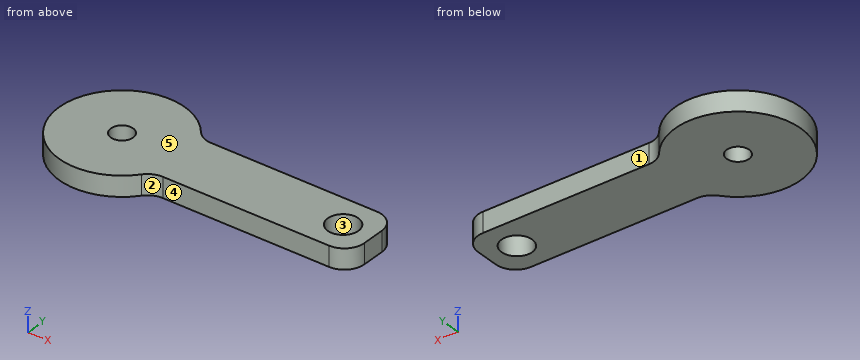
from build123d import *

# Parameters (mm, degrees)
BOSS_EXTRUDE1_DEPTH   = 1.6002
F_0_CLEARANCE_HOLE1_D = 1.778
F_2_CLEARANCE_HOLE1_D = 2.4384


with BuildPart() as part:
    # Sketch1 → Boss-Extrude1 (new body)
    with BuildSketch(Plane.XY):
        with BuildLine():
            Line((5.16599458, -2.5), (18.4125, -2.5))
            ThreePointArc((18.4125, -2.5), (19.535032015, -2.035032015), (20, -0.9125))
            Line((20, -0.9125), (20, 0.9125))
            ThreePointArc((20, 0.9125), (19.535032015, 2.035032015), (18.4125, 2.5))
            Line((18.4125, 2.5), (5.16599458, 2.5))
            ThreePointArc((5.16599458, 2.5), (4.474468718, 2.658532459), (3.921058505, 3.102466793))
            ThreePointArc((3.921058505, 3.102466793), (-5, 0), (3.921058505, -3.102466793))
            ThreePointArc((3.921058505, -3.102466793), (4.474468718, -2.658532459), (5.16599458, -2.5))
        make_face()
    extrude(amount=BOSS_EXTRUDE1_DEPTH)

    # #0 Clearance Hole1 (through all)
    with Locations(Plane.XY.offset(1.6002)):
        with Locations((0, 0)):
            Hole(F_0_CLEARANCE_HOLE1_D / 2)

    # #2 Clearance Hole1 (through all)
    with Locations(Plane.XY.offset(1.6002)):
        with Locations((17.615594793, 0)):
            Hole(F_2_CLEARANCE_HOLE1_D / 2)


solid = part.part
Could you check a few things on this model? Use its own coordinates, in mm. Face numbers are marked on the shaded views. A direction names the side the tool comes from. Give positions to 0.01 mm unless a question says otherwise; leave off trailing zeros. Write each loop counter-clockwise with the first axis right and the second up, starting at its lowest first coordinate (ties: lowest second). Pieces come first, ordered by that corner, then holes. Notation, with made-up numbers: (40, 82.25) - (67, 82.25) arc R15 ccw to (67, 93.25) - close; hole circle Ø10 at (9, 45). An arc over 180 degrees is marked (long way). Use CSV: the item, a comma, the result in double quotes. Start each with the question number.
Item 1: I want a section at D-D, the plane y = -4. Please give me the cut outline in (x, z), then the cut area to 3 significant figures.
Item 2: I want a section at B-B, the plane y = 0. Please give me the cut outline in (x, z), then the cut area to 3 significant figures.
Item 3: I want a section at A-A, the plane x = 0. Please give me the cut outline in (y, z).
Item 4: If I drill on line 1 along Y through (x, z) = (0, 0.6); line 2 along X through (y, z) = (0.75, 1.3); line 3 along X through (y, z) = (-0.25, 0.25), over which ranges is the centre line in solid material (lowest first)?
Item 5: I want a section at C-C, the plane z = 0.4. Please give me the cut outline in (x, y) (1 decimal), then the cut area to 3 significant figures.
Item 6: If we mould it in two halves opening along Y, with no side actions, what happens to the marked faces 1, 2 and 3? For each: pulls with the +Y half, pulls with the -Y half, needs draft (parallel to the pull), parting line crosses it, or undercut.
Item 7: For the marked faces 4 and 5, which set-ups out of +Z, -Z, +X, -X, +Y, -Y let a thin tool reach every point of the face, with its end or its side?
Item 8: I'm going to push a flat-ended pin straight in: pin 1 (1.4 mm diameter, centred on x = 0, y = 0, fed in from -Z). Where does the tip first touch, or does it pass through?
Findings:
1,outline,"(-3, 0) - (3, 0) - (3, 1.6) - (-3, 1.6) - close"
1,area,"9.60 mm2"
2,outline,"(-5, 0) - (-0.89, 0) - (-0.89, 1.6) - (-5, 1.6) - close; (0.89, 0) - (16.4, 0) - (16.4, 1.6) - (0.89, 1.6) - close; (18.83, 0) - (20, 0) - (20, 1.6) - (18.83, 1.6) - close"
2,area,"33.3 mm2"
3,outline,"(-5, 0) - (-0.89, 0) - (-0.89, 1.6) - (-5, 1.6) - close; (0.89, 0) - (5, 0) - (5, 1.6) - (0.89, 1.6) - close"
4,line 1,"y = -5 to -0.89, 0.89 to 5"
4,line 2,"x = -4.94 to -0.48, 0.48 to 16.65, 18.58 to 20"
4,line 3,"x = -4.99 to -0.85, 0.85 to 16.42, 18.81 to 20"
5,outline,"(3.9, -3.1) arc R1.6 cw to (5.2, -2.5) - (18.4, -2.5) arc R1.6 ccw to (20, -0.9) - (20, 0.9) arc R1.6 ccw to (18.4, 2.5) - (5.2, 2.5) arc R1.6 cw to (3.9, 3.1) arc R5 ccw (long way) to start; hole circle Ø1.8 at (0, 0); hole circle Ø2.4 at (17.6, 0)"
5,area,"147 mm2"
6,face 1,"pulls with the +Y half"
6,face 2,"pulls with the -Y half"
6,face 3,"undercut"
7,face 4,"+Z, -Z, +X, -Y"
7,face 5,"+Z, +X, -X, +Y, -Y"
8,pin 1,"passes through"
